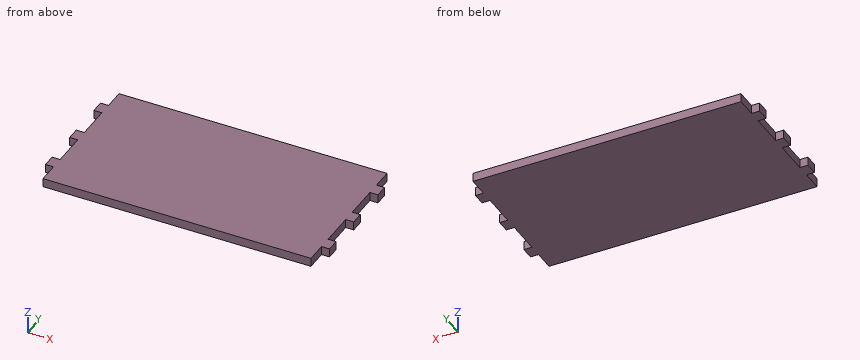
```python
from build123d import *

# Parameters (mm, degrees)
F0_W     = 200
F0_H     = 110
F1_DEPTH = 6.5
F3_DEPTH = 6
F5_DEPTH = 6


with BuildPart() as f1:
    # F0 (on Top) → F1 (new body)
    with BuildSketch(Plane.XY):
        Rectangle(F0_W, F0_H)
    extrude(amount=F1_DEPTH)

    # F2 (on face) → F3 (join)
    with BuildSketch(Plane(origin=(-100, 0, 0), x_dir=(0, -1, 0), z_dir=(-1, 0, 0))):
        Polygon((-39.75, 6.5), (-39.75, 3.25), (-35, 3.25), (-30.25, 3.25), (-30.25, 6.5), align=None)
        Polygon((-35, 3.25), (-39.75, 3.25), (-39.75, 0), (-30.25, 0), (-30.25, 3.25), align=None)
        Polygon((-4.75, 6.5), (-4.75, 3.25), (0, 3.25), (4.75, 3.25), (4.75, 6.5), align=None)
        Polygon((0, 3.25), (-4.75, 3.25), (-4.75, 0), (4.75, 0), (4.75, 3.25), align=None)
        Polygon((39.75, 6.5), (30.25, 6.5), (30.25, 3.25), (35, 3.25), (39.75, 3.25), align=None)
        Polygon((30.25, 3.25), (30.25, 0), (39.75, 0), (39.75, 3.25), (35, 3.25), align=None)
    extrude(amount=F3_DEPTH)

    # F4 (on face) → F5 (join)
    with BuildSketch(Plane.YZ.offset(100)):
        Polygon((-39.75, 6.5), (-39.75, 3.25), (-35, 3.25), (-30.25, 3.25), (-30.25, 6.5), align=None)
        Polygon((-35, 3.25), (-39.75, 3.25), (-39.75, 0), (-30.25, 0), (-30.25, 3.25), align=None)
        Polygon((-4.75, 6.5), (-4.75, 3.25), (0, 3.25), (4.75, 3.25), (4.75, 6.5), align=None)
        Polygon((0, 3.25), (-4.75, 3.25), (-4.75, 0), (4.75, 0), (4.75, 3.25), align=None)
        Polygon((39.75, 6.5), (30.25, 6.5), (30.25, 3.25), (30.25, 0), (39.75, 0), align=None)
    extrude(amount=F5_DEPTH)


solid = f1.part
```
Build history of the part. All positions in model axes, mm. Round coordinates to 2 decimals unless told otherwise and drop trailing zeros. Loops run counter-clockwise (first coordinate to the right, second up) from the corner with the lowest first, then second, coordinate; pieces in that order, holes last.
Item 1: Drill centre line: line 1 along X through (y, z) = (-47.5, 4.75). Where is it in solid material? Low to high.
Item 2: Pin check, flat tips, straight feed: P1, Ø1.8, axis at x = -103.5, z = 2.5, coming from the -Y side; P2, Ø3, axis at y = -45, z = 4, coming from the +X side; P3, Ø2, axis at y = 49, z = 2, coming from the -X side. Stop position of each tip, or through.
Item 3: Saw through at B-B (y = -15). List the corners of the cut face in (x, z).
Item 4: Saw through at A-A (z = 4.75). List the corners of the cut face in (x, y), then the cut area to 3 significant figures.
Worked answers:
1. line 1: x = -100 to 100
2. P1: stops at y = -39.75
2. P2: stops at x = 100
2. P3: stops at x = -100
3. outline: (-100, 0) - (100, 0) - (100, 6.5) - (-100, 6.5) - close
4. outline: (-106, -39.75) - (-100, -39.75) - (-100, -55) - (100, -55) - (100, -39.75) - (106, -39.75) - (106, -30.25) - (100, -30.25) - (100, -4.75) - (106, -4.75) - (106, 4.75) - (100, 4.75) - (100, 30.25) - (106, 30.25) - (106, 39.75) - (100, 39.75) - (100, 55) - (-100, 55) - (-100, 39.75) - (-106, 39.75) - (-106, 30.25) - (-100, 30.25) - (-100, 4.75) - (-106, 4.75) - (-106, -4.75) - (-100, -4.75) - (-100, -30.25) - (-106, -30.25) - close
4. area: 22,300 mm2
